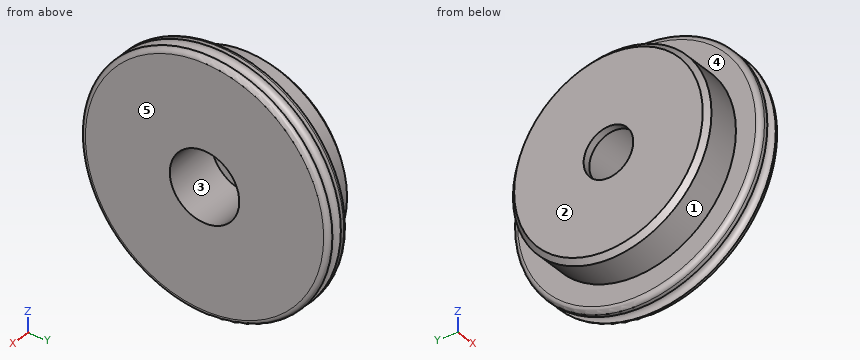
Autodesk Inventor part; units mm, degrees
ref_plane "YZ Plane" through (0, 0, 0) normal (1, 0, 0) x (0, 1, 0)
ref_plane "XZ Plane" through (0, 0, 0) normal (0, 1, 0) x (-1, 0, 0)
ref_plane "XY Plane" through (0, 0, 0) normal (0, 0, 1) x (1, 0, 0)
sketch "Sketch1" plane through (0, 0, 0) normal (0, 0, 1) x (1, 0, 0)
  line L0 (0, 0) -> (25, 0)
  line L1 (25, 0) -> (25, 50)
  line L2 (15, 50) -> (15, 40)
  line L3 (15, 40) -> (0, 40)
  line L4 (0, 40) -> (0, 0)
  line L5 (15, 50) -> (18.5, 50)
  line L6 (18.5, 50) -> (18.5, 47)
  line L7 (18.5, 47) -> (23, 47) construction
  line L8 (23, 47) -> (23, 50)
  line L9 (23, 50) -> (25, 50)
  circle A0 centre (20.75, 50) radius 2.25 construction
  line L10 (18.5, 50) -> (23, 50) construction
  arc A1 (18.5, 50) -> (23, 50) centre (20.75, 50) ccw
  point P0 (23, 48.5)
  point P1 (20.75, 50)
  dimension "d1" = 40
  dimension "d2" = 15
  dimension "d3" = 10
  dimension "d5" = 50
  dimension "d6" = 3
  dimension "d7" = 4.5
  dimension "d8" = 2
revolve "Revolution1" add sketch "Sketch1" angle 360 about axis through (0, 0, 0) along (1, 0, 0)
fillet "Fillet2" radius 2 1 edges at (15, -50, 0)
fillet "Fillet3" radius 2 1 edges at (25, -50, 0)
chamfer "Chamfer1" distance 2 angle 45 1 edges at (0, -40, 0)
sketch "Sketch2" plane through (25, 0, 0) normal (1, 0, 0) x (0, 0, -1)
  circle A0 centre (0, 0) radius 48
hole "Hole1" at (25, 0, 0) direction (-1, 0, 0) diameter 20 end through all
sketch "Sketch3" plane through (25, 0, 0) normal (1, 0, 0) x (0, 0, -1)
  circle A0 centre (0, 0) radius 10
  circle A1 centre (0, 0) radius 48
hole "Hole2" at (25, 0, 0) direction (-1, 0, 0) diameter 28 depth 22
properties part number "P302" material "Aluminum 6061"
Source: CAD feature listing. Evaluate the final solid. Frame: model axes, mm. Face numbers are marked on the shaded views. A direction names the side the tool comes from. Coordinates: 2 decimals unless noted, no trailing zeros. Write each loop counter-clockwise with the first axis right and the second up, starting at its lowest first coordinate (ties: lowest second). Pieces come first, ordered by that corner, then holes. Notation, with made-up numbers: M 74,-9 L 114,-9 A23 ccw 114,10 Z; hole C 51.5,-37.5 d9. An arc over 180 degrees is marked long. Use a Markdown table: item, result.
1) Mould query, pull axis Y, two halves, no side actions, for the marked faces 1, 2 and 3. Classes: pulls with the +Y half, pulls with the -Y half, needs draft (parallel to the pull), parting line crosses it, or undercut.
Conclusion:
| item | result |
|---|---|
| face 1 | parting line crosses it |
| face 2 | needs draft |
| face 3 | undercut |
2) First-contact query: pin 1 Ø3 at (x, z) = (7, -29.5) entering from -Y; pin 2 Ø8 at (x, z) = (8.5, -18.5) entering from -Y; pin 3 Ø17 at (y, z) = (0, 0) entering from -X; pin 4 Ø4 at (x, z) = (19.5, -16.5) entering from -Y. Flat tips, straight axial feed; report the tip coordinate or a pass-through.
Conclusion:
| item | result |
|---|---|
| pin 1 | stops at y = -28.57 |
| pin 2 | stops at y = -37.28 |
| pin 3 | passes through |
| pin 4 | stops at y = -47.77 |
3) Reachability of the marked faces 4 and 5 from +Z, -Z, +X, -X, +Y, -Y: full face, straight path, thin tool, end or side. Return the list, or none.
Conclusion:
| item | result |
|---|---|
| face 4 | -X |
| face 5 | +Z, -Z, +X, +Y, -Y |
4) Section C-C, the plane x = 10.25. Output: boundary loops of the cut face in (y, z), then the cut area to 3 significant figures.
Conclusion:
| item | result |
|---|---|
| outline | C 0,0 d80; hole C 0,0 d28 |
| area | 4,410 mm^2 |
5) Ray query, L1, parallel to Z at x = 2.05, y = 0; L2, parallel to Z at x = 17.75, y = 0; L3, parallel to Y at x = 15.25, z = 1.5. Return the intervals inside material, ascending.
Conclusion:
| item | result |
|---|---|
| L1 | z = -40 to -10, 10 to 40 |
| L2 | z = -50 to -14, 14 to 50 |
| L3 | y = -48.95 to -13.92, 13.92 to 48.95 |
